```python
from build123d import *

# Parameters (mm, degrees)
CROQUIS2_R              = 7.5
CORTAR_EXTRUIR1_DEPTH   = 100
CROQUIS3_W              = 6.941059202
CROQUIS3_H              = 10
CROQUIS3_W_2            = 21.058940798
SALIENTE_EXTRUIR1_DEPTH = 2
CROQUIS4_W              = 28
CROQUIS4_H              = 10
CORTAR_EXTRUIR2_DEPTH   = 2
SALIENTE_EXTRUIR2_DEPTH = 2
SALIENTE_EXTRUIR3_DEPTH = 2
CROQUIS8_R              = 2.5
SALIENTE_EXTRUIR4_DEPTH = 19.5
CROQUIS9_R              = 2.5
CROQUIS9_R_2            = 1
CORTAR_EXTRUIR3_DEPTH   = 6
CROQUIS10_R             = 0.803973648
CORTAR_EXTRUIR4_DEPTH   = 16
CROQUIS11_R             = 7.5
CORTAR_EXTRUIR5_DEPTH   = 86
CROQUIS12_R             = 2
CORTAR_EXTRUIR7_DEPTH   = 86
CROQUIS14_R             = 2
CORTAR_EXTRUIR8_DEPTH   = 86
SALIENTE_EXTRUIR5_DEPTH = 1
ESCALA1_SCALE           = 7


with BuildPart() as part:
    # Croquis1 → Revolución2 (revolve)
    with BuildSketch(Plane.XY, mode=Mode.PRIVATE) as revoluci_n2_sk:
        Polygon((-10.529470399, 0), (-7.5, 0.5), (0, 0.5), (0, 39.5), (-7.5, 39.5), (-10.529470399, 40), (-12.5, 40), (-12.5, 38), (-10.529470399, 38), (-10.529470399, 35.7), (-12.5, 35.7), (-12.5, 33.7), (-10.529470399, 33.7), (-10.529470399, 31.4), (-12.5, 31.4), (-12.5, 29.4), (-10.529470399, 29.4), (-10.529470399, 27.1), (-12.5, 27.1), (-12.5, 25.1), (-10.529470399, 25.1), (-10.529470399, 22.8), (-12.5, 22.8), (-12.5, 20.8), (-10.529470399, 20.8), (-10.529470399, 19.2), (-12.5, 19.2), (-12.5, 17.2), (-10.529470399, 17.2), (-10.529470399, 14.9), (-12.5, 14.9), (-12.5, 12.9), (-10.529470399, 12.9), (-10.529470399, 10.6), (-12.5, 10.6), (-12.5, 8.6), (-10.529470399, 8.6), (-10.529470399, 6.3), (-12.5, 6.3), (-12.5, 4.3), (-10.529470399, 4.3), (-10.529470399, 2), (-12.5, 2), (-12.5, 0), align=None)
    revolve(revoluci_n2_sk.sketch.rotate(Axis((0, 0.5, 0), (0, 1, 0)), 270), axis=Axis((0, 0.5, 0), (0, 1, 0)))

    # Croquis2 → Cortar-Extruir1 (cut)
    with BuildSketch(Plane(origin=(0, 39.5, 0), x_dir=(1, 0, 0), z_dir=(0, 1, 0))):
        with Locations(Location((0, 0, 0), (0, 0, 270))):
            Circle(CROQUIS2_R)
    extrude(amount=-CORTAR_EXTRUIR1_DEPTH, mode=Mode.SUBTRACT)

    # Croquis3 → Saliente-Extruir1 (add)
    with BuildSketch(Plane.XY.offset(10.529470399)):
        with Locations((-14, 20)):
            Rectangle(CROQUIS3_W, CROQUIS3_H)
        with Locations((0, 20)):
            Rectangle(CROQUIS3_W_2, CROQUIS3_H)
    extrude(amount=-SALIENTE_EXTRUIR1_DEPTH)

    # Croquis4 → Cortar-Extruir2 (cut)
    with BuildSketch(Plane.XY.offset(10.529470399)):
        with Locations((-3.470529601, 20)):
            Rectangle(CROQUIS4_W, CROQUIS4_H)
    extrude(amount=CORTAR_EXTRUIR2_DEPTH, mode=Mode.SUBTRACT)

    # Croquis5 → Saliente-Extruir2 (add)
    with BuildSketch(Plane(origin=(10.529470399, 0, 0), x_dir=(0, 0, -1), z_dir=(1, 0, 0))):
        Polygon((-8.529470399, 25), (-2.889330359, 25), (-3.068508508, 15), (-8.411275116, 15), (-8.529470399, 15), align=None)
    extrude(amount=-SALIENTE_EXTRUIR2_DEPTH)

    # Croquis7 → Saliente-Extruir3 (add)
    with BuildSketch(Plane(origin=(0, 25, 0), x_dir=(1, 0, 0), z_dir=(0, 1, 0))):
        with BuildLine():
            Line((10.529470399, -10.529470399), (10.529470399, -17.029470399))
            ThreePointArc((10.529470399, -17.029470399), (7.029470399, -20.529470399), (3.529470399, -17.029470399))
            Line((3.529470399, -17.029470399), (3.529470399, -10.529470399))
            Line((3.529470399, -10.529470399), (10.529470399, -10.529470399))
        make_face()
    extrude(amount=-SALIENTE_EXTRUIR3_DEPTH)

    # Croquis8 → Saliente-Extruir4 (add)
    with BuildSketch(Plane(origin=(0, 0, 0), x_dir=(0, 0, -1), z_dir=(1, 0, 0))):
        with Locations(Location((0, 20, 0), (0, 0, 161.337082109))):
            Circle(CROQUIS8_R)
    extrude(amount=SALIENTE_EXTRUIR4_DEPTH)

    # Croquis9 → Cortar-Extruir3 (cut)
    with BuildSketch(Plane(origin=(19.5, 0, 0), x_dir=(0, 0, -1), z_dir=(1, 0, 0))):
        with Locations(Location((0, 20, 0), (0, 0, 161.337082109))):
            Circle(CROQUIS9_R)
        with Locations((0, 20)):
            Circle(CROQUIS9_R_2, mode=Mode.SUBTRACT)
    extrude(amount=-CORTAR_EXTRUIR3_DEPTH, mode=Mode.SUBTRACT)

    # Croquis10 → Cortar-Extruir4 (cut)
    with BuildSketch(Plane(origin=(19.5, 0, 0), x_dir=(0, 0, -1), z_dir=(1, 0, 0))):
        with Locations((0, 20)):
            Circle(CROQUIS10_R)
    extrude(amount=-CORTAR_EXTRUIR4_DEPTH, mode=Mode.SUBTRACT)

    # Croquis11 → Cortar-Extruir5 (cut)
    with BuildSketch(Plane(origin=(0, 40, 0), x_dir=(1, 0, 0), z_dir=(0, 1, 0))):
        with Locations(Location((0, 0, 0), (0, 0, 270))):
            Circle(CROQUIS11_R)
    extrude(amount=-CORTAR_EXTRUIR5_DEPTH, mode=Mode.SUBTRACT)

    # Croquis12 → Cortar-Extruir7 (cut)
    with BuildSketch(Plane.XY.offset(10.529470399)):
        with Locations((-14.470529601, 18.5)):
            Circle(CROQUIS12_R)
    extrude(amount=-CORTAR_EXTRUIR7_DEPTH, mode=Mode.SUBTRACT)

    # Croquis14 → Cortar-Extruir8 (cut)
    with BuildSketch(Plane.XZ.offset(-23)):
        with Locations(Location((7.529470399, 14.529470399, 0), (0, 0, 270))):
            Circle(CROQUIS14_R)
    extrude(amount=-CORTAR_EXTRUIR8_DEPTH, mode=Mode.SUBTRACT)

    # Croquis15 → Saliente-Extruir5 (add)
    with BuildSketch(Plane(origin=(0, 20, 0), x_dir=(-1, 0, 0), z_dir=(0, -1, 0))):
        with BuildLine():
            Line((-6.835484568, -3.086446293), (-6.835484568, 3.086446293))
            ThreePointArc((-6.835484568, 3.086446293), (-7.5, 0), (-6.835484568, -3.086446293))
        make_face()
    extrude(amount=-SALIENTE_EXTRUIR5_DEPTH)


with BuildPart() as part_1:
    # Escala1: scaled about (0.011645774, 20.045435338, 0.404795785)
    add(part.part.scale(ESCALA1_SCALE).moved(Location((-0.069874644, -120.272612028, -2.42877471))))


solid = part_1.part
```
For this review, take the finished solid that the model builds, in its own axes (mm). A direction names the side the tool comes from. Give positions to 0.01 mm unless a question says otherwise; leave off trailing zeros. Order: outer loops, then holes, each group sorted by start corner. A loop starts at its lowest first (then second) coordinate and runs counter-clockwise, first axis right, second up.
1) Take a section at B-B (z = 123). Give the boundary of the cut face in (x, y), then the cut area to 3 significant figures.
2) Take a section at A-A (y = -69). Give the boundary of the cut face in (x, z), then the cut area to 3 significant figures.
3) For faces 1 (the face through (-26, 62, -86)), 2 (the face through (51.93, 19.65, 49.81)), 3 (the face through (136.43, 15, -6)), 4 (the face through (59, -15.273, 59)), list the 3-axis set-ups (+Z, -Z, +X, -X, +Y, -Y) from which the entire face can be reached by the end or side of a thin tool; tool diameter is ignored.
4) Insertion check: pin 1 (5.5 mm diameter, centred on y = 23.5, z = 8, fed in from -X); pin 2 (1 mm diameter, centred on x = -56, y = 128.5, fed in from -Z); pin 3 (5 mm diameter, centred on y = 38, z = 105.5, fed in from +X); pin 4 (5 mm diameter, centred on y = -81.5, z = -66, fed in from +X). Each pin has a flat end and moves straight along its axis. Give the tip position at first contact, or say it passes through.
5) Wall thickness on line 1 (Z direction, x = 1, y = 102); line 2 (X direction, y = 37.5, z = -47.5); line 3 (Y direction, x = -52, z = -54.5): over which ranges is each line inside the solid? List them lowest first.
6) The part is to be moulded in two halves that separate along Y. For faces 5 (the face through (49.68, 47.83, 141.27)), 6 (the face through (44.78, 137.56, 56.06)), say which applies: released by +Y, released by -Y, zero draft, split by the parting line, or undercut.
Derived:
1. outline: (25.44, 40.73) - (72.83, 40.73) - (72.83, 54.73) - (25.44, 54.73) - close
1. area: 664 mm2
2. outline: circle Ø147.41 at (-0.07, -2.43); hole circle Ø105 at (-0.07, -2.43)
2. area: 8,410 mm2
3. face 1: +Y
3. face 2: none
3. face 3: +Z, -Z, +X, +Y, -Y
3. face 4: +Z, +X
4. pin 1: stops at x = -87.17
4. pin 2: stops at z = -70.13
4. pin 3: passes through
4. pin 4: stops at x = 62.59
5. line 1: z = -76.13 to -54.92, 50.06 to 71.27
5. line 2: x = -75.07 to -26.99, 26.85 to 74.93
5. line 3: y = -120.25 to 159.7
6. face 5: zero draft
6. face 6: undercut
